Input: dimensioned drawing with shaded views. Units: mm. Origin: part minimum x, y, z. A direction names the side the tool comes from. Round coordinates to 2 decimals unless told otherwise and drop trailing zeros. Order: outer loops, then holes, each group sorted by start corner. A loop starts at its lowest first (then second) coordinate and runs counter-clockwise, first axis right, second up. Notation, with made-up numbers: M 36.25,-6.75 L 48.25,-6.75 A21 cw 48.25,13.25 Z; hole C 63.25,65 d4. An arc over 180 degrees is marked long. Put each result on its own line as item: value. Start each with the question number.
1) Section C-C, the plane y = 1.5. Return loops of the section in (x, z), then the cut area to 3 significant figures.
2) Material intervals for probe 1 along Z at (x, y) = (9.25, 6.75); probe 2 along Z at (x, y) = (9.25, 16.75); probe 3 along Y at (x, z) = (5.5, 11.5), sorted ascending. Write a range as [from, to].
3) First-contact query: P1, Ø8, axis at y = 4, z = 16, coming from the +X side; P2, Ø3, axis at x = 15, y = 11.5, coming from the +Z side; P3, Ø1.5, axis at y = 15.5, z = 15.5, coming from the -X side. Flat tips, straight axial feed; report the tip coordinate or a pass-through.
4) Section B-B, the plane z = 9.25. Return loops of the section in (x, y).
5) Section D-D, the plane x = 16.5. Return loops of the section in (y, z), then the cut area to 3 significant figures.
6) Draft query along Z for the marked faces 3, 4 and 5. Return one class per face: pulls with the +Z half, pulls with the -Z half, needs draft (parallel to the pull), parting line crosses it, or undercut.
7) Access query for the marked faces 1 and 2. Directions: +Z, -Z, +X, -X, +Y, -Y. A direction counts if a zero-diameter tool reaches every point of the face in a straight line with its end or side. Return the directions, or none.
8) Section A-A, the plane x = 9.25. Return loops of the section in (y, z).
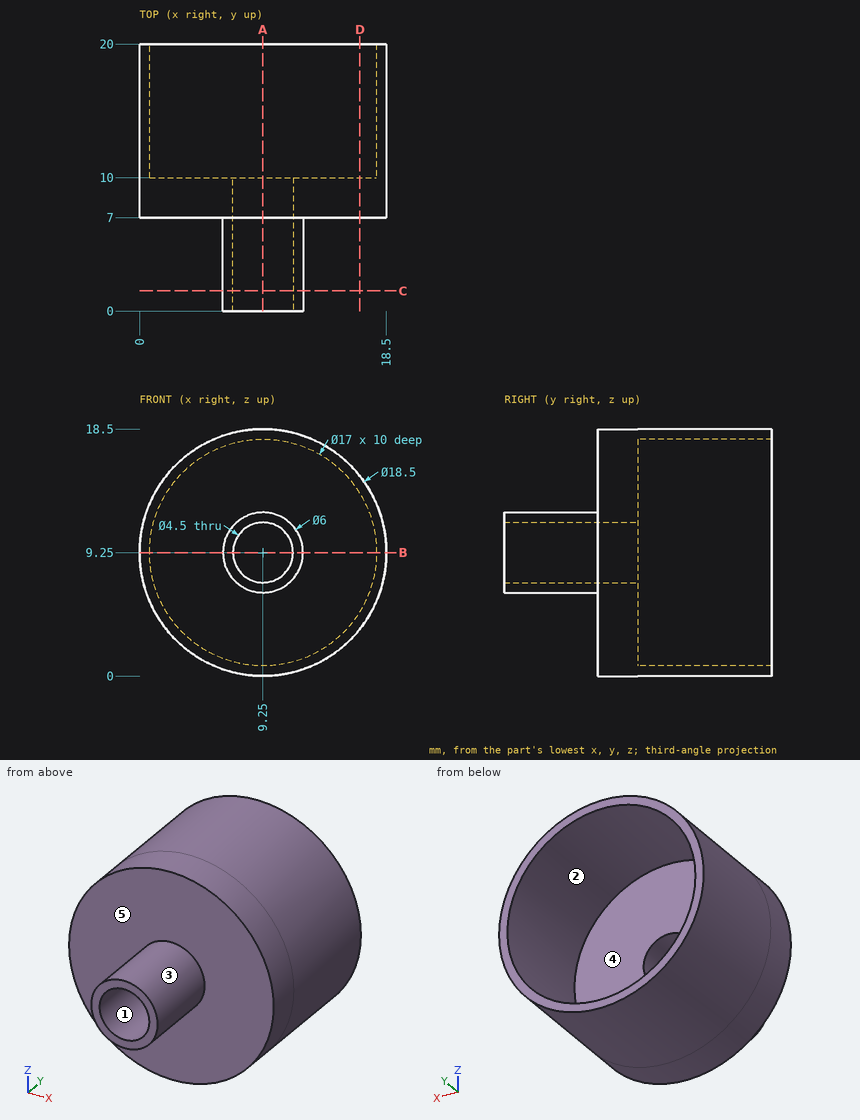
Result sheet:
1. outline: C 9.25,9.25 d6; hole C 9.25,9.25 d4.5
1. area: 12.4 mm2
2. probe 1: z = [6.25, 7], [11.5, 12.25]
2. probe 2: z = [0, 0.75], [17.75, 18.5]
2. probe 3: y = [7, 10]
3. P1: stops at x = 17.54
3. P2: stops at z = 17.47
3. P3: stops at x = 1.81
4. outline: M 0,7 L 6.25,7 L 6.25,0 L 7,0 L 7,10 L 0.75,10 L 0.75,20 L 0,20 Z; M 11.5,0 L 12.25,0 L 12.25,7 L 18.5,7 L 18.5,20 L 17.75,20 L 17.75,10 L 11.5,10 Z
5. outline: M 7,3.51 L 20,3.51 L 20,4.81 L 10,4.81 L 10,13.69 L 20,13.69 L 20,14.99 L 7,14.99 Z
5. area: 60.6 mm2
6. face 3: parting line crosses it
6. face 4: undercut
6. face 5: needs draft
7. face 1: +Y, -Y
7. face 2: +Y
8. outline: M 0,6.25 L 7,6.25 L 7,0 L 20,0 L 20,0.75 L 10,0.75 L 10,7 L 0,7 Z; M 0,11.5 L 10,11.5 L 10,17.75 L 20,17.75 L 20,18.5 L 7,18.5 L 7,12.25 L 0,12.25 Z
